Input: part model. Units: mm. Frame: model coordinates. Face numbers are marked on the shaded views. Coordinates: 2 decimals unless noted, no trailing zeros. Write each loop counter-clockwise with the first axis right and the second up, starting at its lowest first coordinate (ties: lowest second). Pieces come first, ordered by that corner, then holes. Notation, with made-up numbers: (53.25, -29.75) - (80.25, -29.75) arc R26 ccw to (80.25, 4.25) - close; hole circle Ø7 at (-8, 35). An arc over 180 degrees is marked (long way). Put each result on its own line as item: value. Start each with the question number.
1. Cut plane A-A, the plane y = 0. Return loops of the section in (x, z).
2. Pin query (flat end, axial travel): pin 1 (17.5 mm diameter, centred on y = 0, z = 0, fed in from -X). Return the tip coordinate at first contact, or that it passes through.
3. Line query: line 1 (Y direction, x = -4.7, z = 0); line 2 (Y direction, x = -5.35, z = -2.5); line 3 (Z direction, x = -1.25, y = -1). Output: solid intervals per line, ascending.
4. Pull-direction query (Y, two-part tool) for the marked faces 1, 2, 3 and 4; classes: released by +Y, released by -Y, zero draft, split by the parting line, or undercut.
5. Cut plane C-C, the plane x = -5.15. Return loops of the section in (y, z), and give its area (3 significant figures).
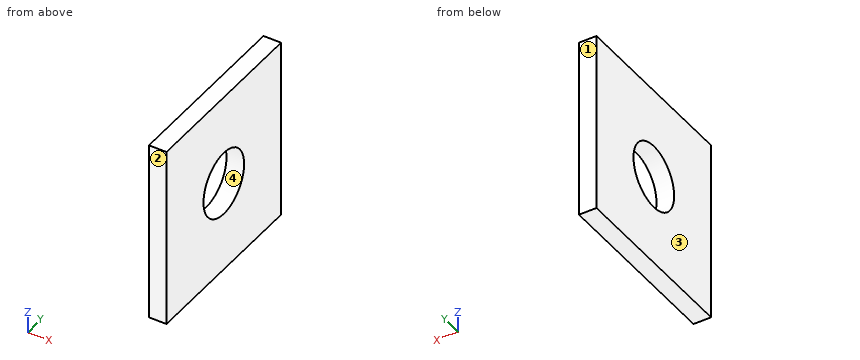
from build123d import *

# Parameters (mm, degrees)
SKETCH1_W  = 62
SKETCH1_H  = 62
SKETCH1_R  = 11
BODY_DEPTH = 6


with BuildPart() as part:
    # Sketch1 → Body (new body)
    with BuildSketch(Plane(origin=(0, 0, 0), x_dir=(0, 0, -1), z_dir=(1, 0, 0))):
        Rectangle(SKETCH1_W, SKETCH1_H)
        Circle(SKETCH1_R, mode=Mode.SUBTRACT)
    extrude(amount=-BODY_DEPTH)


solid = part.part
Report:
1. outline: (-6, -31) - (0, -31) - (0, -11) - (-6, -11) - close; (-6, 11) - (0, 11) - (0, 31) - (-6, 31) - close
2. pin 1: passes through
3. line 1: y = -31 to -11, 11 to 31
3. line 2: y = -31 to -10.71, 10.71 to 31
3. line 3: z = -31 to -10.95, 10.95 to 31
4. face 1: released by +Y
4. face 2: released by -Y
4. face 3: zero draft
4. face 4: undercut
5. outline: (-31, -31) - (31, -31) - (31, 31) - (-31, 31) - close; hole circle Ø22 at (0, 0)
5. area: 3,460 mm^2
